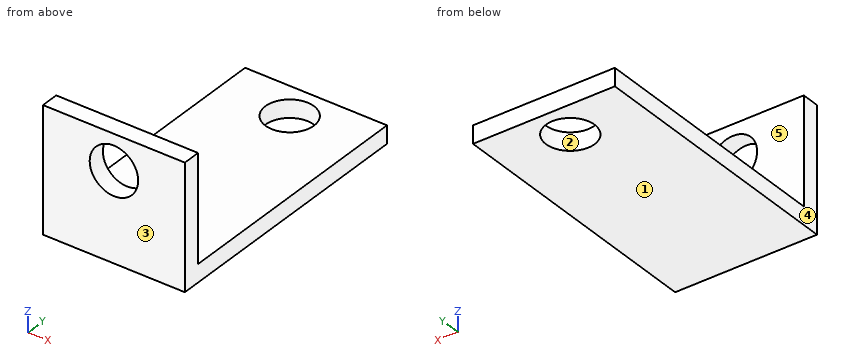
```python
from build123d import *

# Parameters (mm, degrees)
F0_W     = 12
F0_H     = 23
F1_DEPTH = 1.5
F2_R     = 2.05
F3_DEPTH = 25
F4_W     = 12
F4_H     = 1.5
F5_DEPTH = 9
F6_R     = 2.05
F7_DEPTH = 25


with BuildPart() as f1:
    # F0 (on Top) → F1 (new body)
    with BuildSketch(Plane.XY):
        with Locations((-17.322744, 12.958014)):
            Rectangle(F0_W, F0_H)
    extrude(amount=F1_DEPTH)

    # F2 (on face) → F3 (cut)
    with BuildSketch(Plane.XY.offset(1.5)):
        with Locations((-17.322744, 21.458014)):
            Circle(F2_R)
    extrude(amount=-F3_DEPTH, mode=Mode.SUBTRACT)

    # F4 (on face) → F5 (join)
    with BuildSketch(Plane.XY.offset(1.5)):
        with Locations((-17.322744, 2.208014)):
            Rectangle(F4_W, F4_H)
    extrude(amount=F5_DEPTH)

    # F6 (on face) → F7 (cut)
    with BuildSketch(Plane(origin=(0, 2.958014, 0), x_dir=(-1, 0, 0), z_dir=(0, 1, 0))):
        with Locations((17.322744, 7.5)):
            Circle(F6_R)
    extrude(amount=-F7_DEPTH, mode=Mode.SUBTRACT)


solid = f1.part
```
The listing builds one solid part. Answer for the finished solid, in the listing's coordinates (mm). Face numbers are marked on the shaded views. A direction names the side the tool comes from. Give positions to 0.01 mm unless a question says otherwise; leave off trailing zeros. Order: outer loops, then holes, each group sorted by start corner. A loop starts at its lowest first (then second) coordinate and runs counter-clockwise, first axis right, second up. Notation, with made-up numbers: (81, 62.25) -> (132, 62.25) arc R24 cw to (132, 98.25) -> close; hole circle Ø3 at (47.25, -2). An arc over 180 degrees is marked (long way). Answer as CSV lines item,"result". Start each with the question number.
Q1. Given pin 1 (3 mm diameter, centred on x = -22, y = 16.5, fed in from +Z); pin 2 (3 mm diameter, centred on x = -14, z = 4, fed in from +Y), each flat-ended and moving along its own axis, determine where each tip first touches the part or whether it passes through.
Q2. A cutting plane is placed at C-C (x = -14.75). Determine the outline of the cut face in (y, z).
Q3. A cutting plane is placed at D-D (y = 3.5). Determine the outline of the cut face in (x, z).
Q4. Which of the six approach directions +Z, -Z, +X, -X, +Y, -Y give full straight-line access (tool end or side, diameter ignored) to the marked faces 4 and 5?
Q5. A cutting plane is placed at A-A (z = 7.5). Determine the outline of the cut face in (x, y), then the cut area to 4 significant figures.
Q6. Find the intervals of material crossed by L1, parallel to Z at x = -22, y = 10; L2, parallel to Y at x = -20, z = 2, in increasing order.
Q7. A cutting plane is placed at B-B (y = 21.75). Determine the outline of the cut face in (x, z).
Q8. Determine the mould class of the marked faces 1, 2 and 3 for opening direction Y: pulls with the +Y half, pulls with the -Y half, needs draft (parallel to the pull), parting line crosses it, or undercut.
Results found:
1,pin 1,"z = 1.5"
1,pin 2,"y = 2.96"
2,outline,"(1.46, 0) -> (24.46, 0) -> (24.46, 1.5) -> (2.96, 1.5) -> (2.96, 10.5) -> (1.46, 10.5) -> close"
3,outline,"(-23.32, 0) -> (-11.32, 0) -> (-11.32, 1.5) -> (-23.32, 1.5) -> close"
4,face 4,"+Z, -Z, -X, +Y, -Y"
4,face 5,"+Z, +X, -X, +Y"
5,outline,"(-23.32, 1.46) -> (-19.37, 1.46) -> (-19.37, 2.96) -> (-23.32, 2.96) -> close; (-15.27, 1.46) -> (-11.32, 1.46) -> (-11.32, 2.96) -> (-15.27, 2.96) -> close"
5,area,"11.85 mm2"
6,L1,"0 to 1.5"
6,L2,"1.46 to 2.96"
7,outline,"(-23.32, 0) -> (-19.35, 0) -> (-19.35, 1.5) -> (-23.32, 1.5) -> close; (-15.29, 0) -> (-11.32, 0) -> (-11.32, 1.5) -> (-15.29, 1.5) -> close"
8,face 1,"needs draft"
8,face 2,"undercut"
8,face 3,"pulls with the -Y half"
